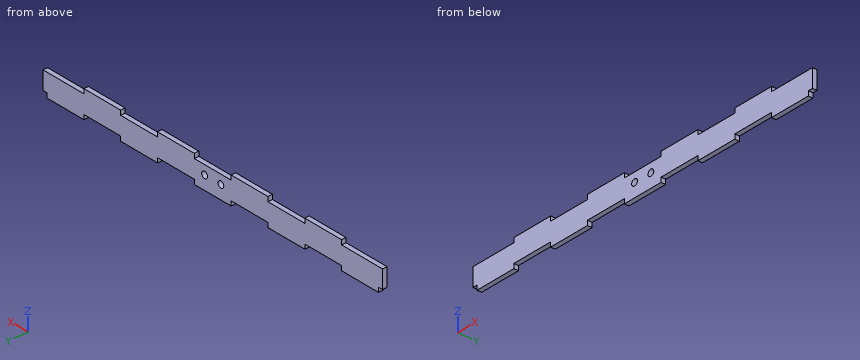
from build123d import *

# Parameters (mm, degrees)
SKETCH1_R           = 2.25
BOSS_EXTRUDE2_DEPTH = 3.175


with BuildPart() as part:
    # Sketch1 → Boss-Extrude2 (new body)
    with BuildSketch(Plane(origin=(0, 0, 0), x_dir=(1, 0, 0), z_dir=(0, 1, 0))):
        Polygon((-128.905, 9.525), (-100.259444444, 9.525), (-100.259444444, 6.35), (-71.613888889, 6.35), (-71.613888889, 9.525), (-42.968333333, 9.525), (-42.968333333, 6.35), (-14.322777778, 6.35), (-14.322777778, 9.525), (14.322777778, 9.525), (14.322777778, 6.35), (42.968333333, 6.35), (42.968333333, 9.525), (71.613888889, 9.525), (71.613888889, 6.35), (100.259444444, 6.35), (100.259444444, 9.525), (128.905, 9.525), (128.905, 6.35), (132.08, 6.35), (132.08, -6.35), (100.259444444, -6.35), (100.259444444, -9.525), (71.613888889, -9.525), (71.613888889, -6.35), (42.968333333, -6.35), (42.968333333, -9.525), (14.322777778, -9.525), (14.322777778, -6.35), (-14.322777778, -6.35), (-14.322777778, -9.525), (-42.968333333, -9.525), (-42.968333333, -6.35), (-71.613888889, -6.35), (-71.613888889, -9.525), (-100.259444444, -9.525), (-100.259444444, -6.35), (-132.08, -6.35), (-132.08, 6.35), (-128.905, 6.35), align=None)
        with Locations((6.35, 0)):
            Circle(SKETCH1_R, mode=Mode.SUBTRACT)
        with Locations((-6.35, 0)):
            Circle(SKETCH1_R, mode=Mode.SUBTRACT)
    extrude(amount=BOSS_EXTRUDE2_DEPTH)


solid = part.part
The model under review builds one solid part; all positions refer to its coordinate system, in mm. Round coordinates to 2 decimals unless told otherwise and drop trailing zeros. Loops run counter-clockwise (first coordinate to the right, second up) from the corner with the lowest first, then second, coordinate; pieces in that order, holes last. Notation, with made-up numbers: (62, -28) - (94, -28) arc R30 cw to (94, 2) - close; hole circle Ø9 at (78.5, 28). An arc over 180 degrees is marked (long way). Use CSV: the item, a comma, the result in double quotes.
(1) Take a section at A-A, the plane x = -6.35. Give the boundary of the cut face in (y, z) (3 decimals), plus the area to 3 significant figures.
Working result:
outline,"(0, -9.525) - (3.175, -9.525) - (3.175, -2.25) - (0, -2.25) - close; (0, 2.25) - (3.175, 2.25) - (3.175, 6.35) - (0, 6.35) - close"
area,"36.1 mm^2"
(2) Take a section at B-B, the plane z = 0. Give the boundary of the cut face in (x, y) (3 decimals).
Working result:
outline,"(-132.08, 0) - (-8.6, 0) - (-8.6, 3.175) - (-132.08, 3.175) - close; (-4.1, 0) - (4.1, 0) - (4.1, 3.175) - (-4.1, 3.175) - close; (8.6, 0) - (132.08, 0) - (132.08, 3.175) - (8.6, 3.175) - close"
(3) For line 1 (X direction, y = 1.35, z = 0); line 2 (X direction, y = 0.9, z = 6.5); line 3 (X direction, y = 0.3, z = -0.5), list the stretches that pass through material, from the lowest coordinate up.
Working result:
line 1,"x = -132.08 to -8.6, -4.1 to 4.1, 8.6 to 132.08"
line 2,"x = -100.26 to -71.61, -42.97 to -14.32, 14.32 to 42.97, 71.61 to 100.26"
line 3,"x = -132.08 to -8.54, -4.16 to 4.16, 8.54 to 132.08"
(4) Clearance check with flat-ended pins moving along their axes: P1, Ø1, axis at y = 2, z = -7.5, coming from the +X side (3 decimals); P2, Ø1.6, axis at x = -131, y = 2.5, coming from the -Z side; P3, Ø4, axis at x = -6.35, z = 0, coming from the +Y side; P4, Ø1, axis at y = 1, z = -7.5, coming from the -X side (3 decimals). State where each tip first meets the part, or that it passes through.
Working result:
P1,"stops at x = 128.905"
P2,"stops at z = -6.35"
P3,"passes through"
P4,"stops at x = -128.905"
